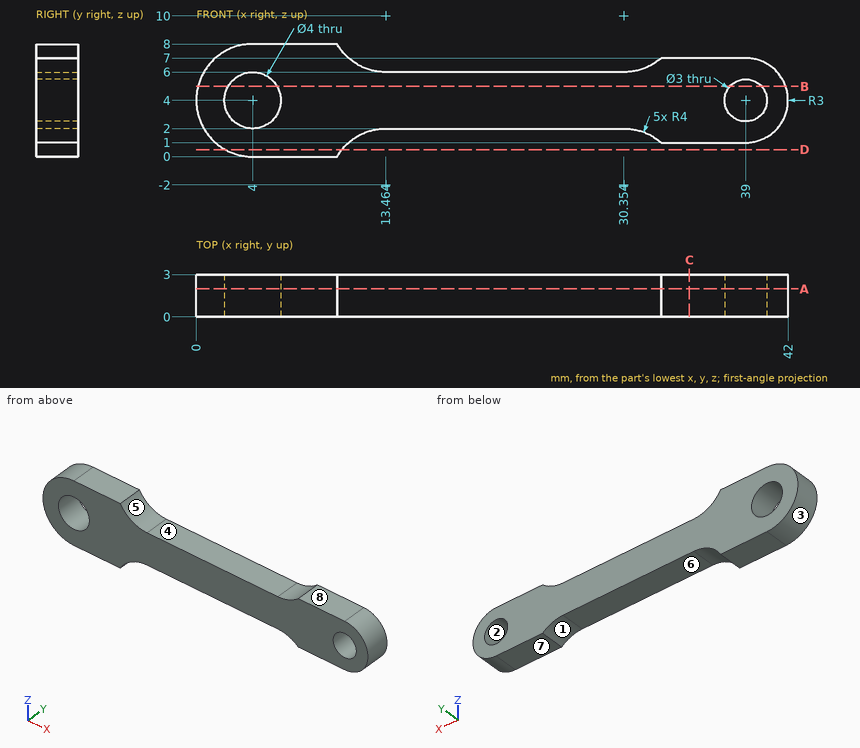
Here's the drawing with two shaded views (mm, measured from the low corner). I have some questions. A direction names the side the tool comes from. Coordinates: 2 decimals unless noted, no trailing zeros. Write each loop counter-clockwise with the first axis right and the second up, starting at its lowest first coordinate (ties: lowest second). Pieces come first, ordered by that corner, then holes.
Item 1: On a 3-axis mill with a long thin cutter (end or side, diameter ignored), from which of +Z, -Z, +X, -X, +Y, -Y can I reach the whole of each face in a straight line? I mean the marked faces 5, 6, 7 and 8. Say none if no direction works.
Item 2: I want a section at D-D on z = 0.5. Write out the boundary of the cut face in (x, y), and give its area (3 significant figures).
Item 3: Will these pins go through, and if not, where does the flat tip stop? pin 1 (0.9 mm diameter, centred on x = 25, y = 2, fed in from -Z); pin 2 (1.8 mm diameter, centred on x = 39, z = 4, fed in from -Y).
Item 4: I want a section at B-B on z = 5. Write out the boundary of the cut face in (x, y), and give its area (3 significant figures).
Item 5: If I drill on line 1 (X direction, y = 1.5, z = 4); line 2 (Z direction, x = 4, y = 1.2); line 3 (X direction, y = 2.8, z = 4.5) (1 decimal), over which ranges is the centre line in solid material (lowest first)?
Item 6: I want a section at A-A on y = 2. Write out the boundary of the cut face in (x, z), and give its area (3 significant figures).
Item 7: I want a section at C-C on x = 35. Write out the boundary of the cut face in (y, z), and give its area (3 significant figures).
Item 8: If we mould it in two halves opening along Z, with no side actions, what happens to the marked faces 1, 2, 3 and 4? For each: +Z half, -Z half, draft (parallel to the pull), parting line (faces both ways), or undercut.
Findings below:
1. face 5: +Z, +Y, -Y
1. face 6: -Z, +Y, -Y
1. face 7: -Z, +X, +Y, -Y
1. face 8: +Z, +X, +Y, -Y
2. outline: (2.06, 0) - (10.34, 0) - (10.34, 3) - (2.06, 3) - close
2. area: 24.8 mm2
3. pin 1: stops at z = 2
3. pin 2: passes through
4. outline: (0.13, 0) - (2.27, 0) - (2.27, 3) - (0.13, 3) - close; (5.73, 0) - (37.88, 0) - (37.88, 3) - (5.73, 3) - close; (40.12, 0) - (41.83, 0) - (41.83, 3) - (40.12, 3) - close
4. area: 108 mm2
5. line 1: x = 0 to 2, 6 to 37.5, 40.5 to 42
5. line 2: z = 0 to 2, 6 to 8
5. line 3: x = 0 to 2.1, 5.9 to 37.6, 40.4 to 42
6. outline: (4, 0) - (10, 0) arc R4 cw to (13.46, 2) - (30.35, 2) arc R4 cw to (33, 1) - (39, 1) arc R3 ccw to (39, 7) - (33, 7) arc R4 cw to (30.35, 6) - (13.46, 6) arc R4 cw to (10, 8) - (4, 8) arc R4 ccw to start; hole circle Ø4 at (4, 4); hole circle Ø3 at (39, 4)
6. area: 201 mm2
7. outline: (0, 1) - (3, 1) - (3, 7) - (0, 7) - close
7. area: 18.0 mm2
8. face 1: -Z half
8. face 2: undercut
8. face 3: parting line
8. face 4: +Z half
